Here's the drawing with two shaded views (mm, measured from the low corner). I have some questions. A direction names the side the tool comes from. Give positions to 0.01 mm unless a question says otherwise; leave off trailing zeros. Write each loop counter-clockwise with the first axis right and the second up, starting at its lowest first coordinate (ties: lowest second). Pieces come first, ordered by that corner, then holes. Notation, with made-up numbers: M -1,7.25 L 44,7.25 A21 cw 44,46.25 Z; hole C 18,85 d10. An arc over 180 degrees is marked long. Answer as a JSON object with one key per item and string values. Group by question number.
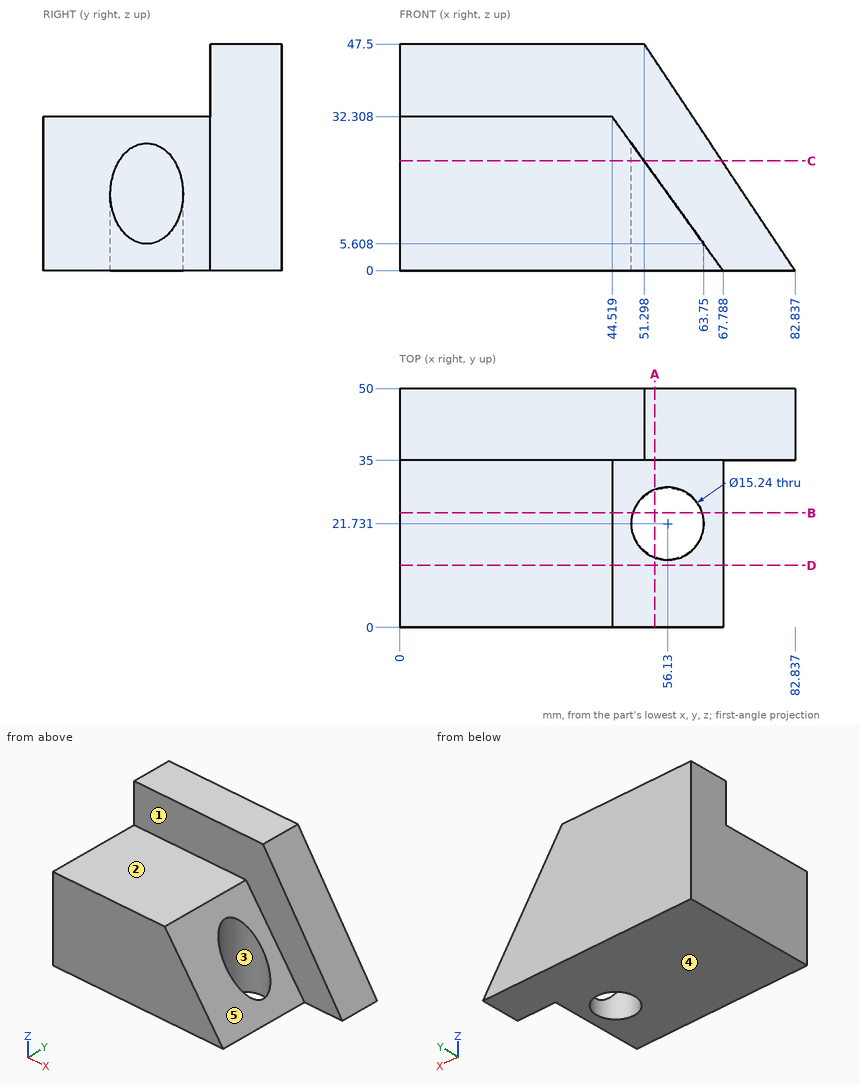
1) We'd pull the mould along Y, two halves only. Please class the marked faces 1, 2 and 3: released by +Y, released by -Y, zero draft, split by the parting line, or undercut.
2) If we section it at B-B, the plane y = 24: List the corners of the cut face in (x, z) for me (1 decimal), plus the area to 3 significant figures.
3) Please list where these lines run through material, in increasing order: line 1 along Y through (x, z) = (20.5, 38.5); line 2 along Z through (x, y) = (40, 6); line 3 along Y through (x, z) = (51, 22.5) (1 decimal). Write a range as from..to.
4) If we section it at A-A, the plane x = 53.5: List the corners of the cut face in (y, z) for me, plus the area to 3 significant figures.
5) I'm going to push flat-ended pins straight in: pin 1 (10.5 mm diameter, centred on x = 14, y = 25.5, fed in from +Z); pin 2 (8 mm diameter, centred on y = 13.5, z = 11, fed in from +X); pin 3 (12 mm diameter, centred on x = 56.13, y = 21.73, fed in from -Z); pin 4 (8 mm diameter, centred on x = 72.5, z = 6.5, fed in from -Y). Where does each tip first touch, or does it pass through?
6) For the marked faces 4 and 5, which set-ups out of +Z, -Z, +X, -X, +Y, -Y let a thin tool reach every point of the face, with its end or its side?
7) If we section it at C-C, the plane z = 23: List the corners of the cut face in (x, y) for me (1 decimal).
8) If we section it at D-D, the plane y = 13: List the corners of the cut face in (x, z) for me, plus the area to 3 significant figures.
Taken from the geometry:
{
 "1": {"face 1": "released by -Y", "face 2": "zero draft", "face 3": "undercut"},
 "2": {"outline": "M 0,0 L 48.9,0 L 48.9,26.3 L 44.5,32.3 L 0,32.3 Z; M 63.4,0 L 67.8,0 L 63.4,6.1 Z", "area": "1,580 mm²"},
 "3": {"line 1": "35..50", "line 2": "0..32.31", "line 3": "0..16.1, 27.4..50"},
 "4": {"outline": "M 0,0 L 14.58,0 L 14.58,19.84 L 0,19.84 Z; M 28.88,0 L 50,0 L 50,44.18 L 35,44.18 L 35,19.84 L 28.88,19.84 Z", "area": "1,070 mm²"},
 "5": {"pin 1": "z = 32.31", "pin 2": "x = 62.75", "pin 3": "through", "pin 4": "y = 35"},
 "6": {"face 4": "-Z, +X, -X, +Y, -Y", "face 5": "+Z, +X, -Y"},
 "7": {"outline": "M 0,0 L 51.2,0 L 51.2,15.9 A7.6 cw 51.2,27.6 L 51.2,35 L 67.6,35 L 67.6,50 L 0,50 Z"},
 "8": {"outline": "M 0,0 L 67.79,0 L 44.52,32.31 L 0,32.31 Z", "area": "1,810 mm²"}
}
